```python
from build123d import *

# Parameters (mm, degrees)
EXTRUDE_1_DEPTH     = 6
SKETCH_2_R          = 1.5
CUT_EXTRUDE_1_DEPTH = 3
SKETCH_3_R          = 1.5
EXTRUDE_2_DEPTH     = 6


with BuildPart() as part:
    # 草图1 → 凸台-拉伸1 (new body)
    with BuildSketch(Plane.XY):
        Polygon((2.713546265, 0), (1.356773133, 2.35), (-1.356773133, 2.35), (-2.713546265, 0), (-1.356773133, -2.35), (1.356773133, -2.35), align=None)
    extrude(amount=-EXTRUDE_1_DEPTH)

    # 草图2 → 切除-拉伸1 (cut)
    with BuildSketch(Plane.XY):
        Circle(SKETCH_2_R)
    extrude(amount=-CUT_EXTRUDE_1_DEPTH, mode=Mode.SUBTRACT)

    # 草图3 → 凸台-拉伸2 (add)
    with BuildSketch(Plane(origin=(0, 0, -6), x_dir=(-1, 0, 0), z_dir=(0, 0, -1))):
        with Locations(Location((0, 0, 0), (0, 0, 180))):
            Circle(SKETCH_3_R)
    extrude(amount=EXTRUDE_2_DEPTH)


solid = part.part
```
Part model, mm, in its own coordinate system. A direction names the side the tool comes from. Round coordinates to 2 decimals unless told otherwise and drop trailing zeros. Write each loop counter-clockwise with the first axis right and the second up, starting at its lowest first coordinate (ties: lowest second). Pieces come first, ordered by that corner, then holes. Notation, with made-up numbers: M 42.25,30.25 L 53.25,30.25 A16 cw 53.25,60.25 Z; hole C 64.5,56.5 d10. An arc over 180 degrees is marked long. Answer as CSV lines item,"result". Start each with the question number.
1) Mould opens along Y. For faces 1 (the face through (-1.5, 0.07, -1.48)), 2 (the face through (0, -2.35, -3)), 3 (the face through (-2.026, 1.191, -2.958)) say: +Y half, -Y half, draft (parallel to the pull), parting line (faces both ways), or undercut.
2) Band-saw the part on C-C (y = 1.3). List the corners of the cut face in (x, z), then the cut area to 3 significant figures.
3) Drill centre lines: L1, parallel to Y at x = 0, z = -0.9; L2, parallel to Z at x = 0.65, y = 0.9; L3, parallel to Z at x = 1.5, y = 1.6. Where is each one in solid material? Low to high.
4) Band-saw the part on B-B (z = -5). List the corners of the cut face in (x, y).
5) Band-saw the part on A-A (x = 0). List the corners of the cut face in (y, z).
6) Which spindle directions (+Z, -Z, +X, -X, +Y, -Y) get a long thin tool onto all of the face, cutting with end or side? Do faces 4 (the face through (0, 0, -3)), 5 (the face through (1.43, -0.45, -8.96)), 6 (the face through (-2.045, -1.159, -2.958)). Say none if no direction does.
7) Band-saw the part on D-D (z = -7.75). List the corners of the cut face in (x, y), then the cut area to 3 significant figures.
Worked out:
1,face 1,"undercut"
1,face 2,"-Y half"
1,face 3,"+Y half"
2,outline,"M -1.96,-6 L -0.75,-6 L -0.75,-12 L 0.75,-12 L 0.75,-6 L 1.96,-6 L 1.96,0 L 0.75,0 L 0.75,-3 L -0.75,-3 L -0.75,0 L -1.96,0 Z"
2,area,"28.0 mm²"
3,L1,"-2.35 to -1.5, 1.5 to 2.35"
3,L2,"-12 to -3"
3,L3,"-6 to 0"
4,outline,"M -2.71,0 L -1.36,-2.35 L 1.36,-2.35 L 2.71,0 L 1.36,2.35 L -1.36,2.35 Z"
5,outline,"M -2.35,-6 L -1.5,-6 L -1.5,-12 L 1.5,-12 L 1.5,-6 L 2.35,-6 L 2.35,0 L 1.5,0 L 1.5,-3 L -1.5,-3 L -1.5,0 L -2.35,0 Z"
6,face 4,"+Z"
6,face 5,"-Z"
6,face 6,"+Z, -Z, -X, -Y"
7,outline,"C 0,0 d3"
7,area,"7.07 mm²"
